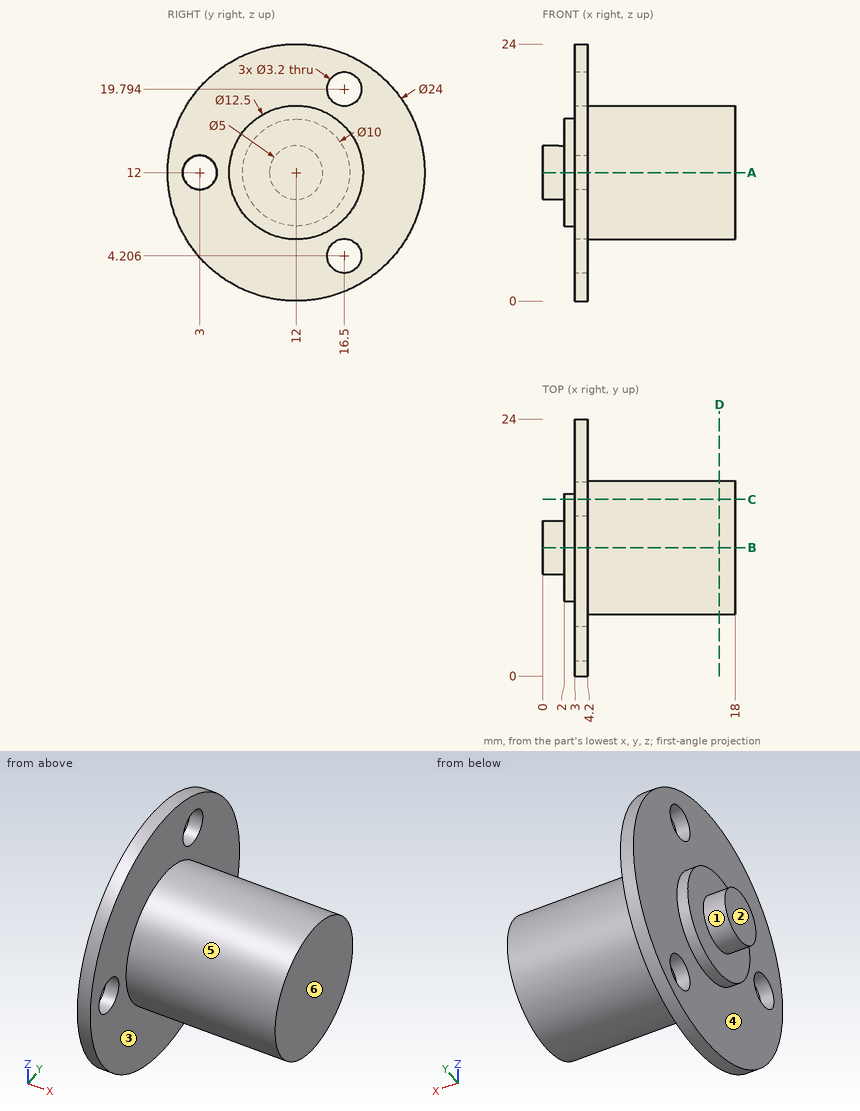
Drawing for the job (mm, zero at the part's lowest x, y, z). A direction names the side the tool comes from. Give positions to 0.01 mm unless a question says otherwise; leave off trailing zeros. Loops run counter-clockwise (first coordinate to the right, second up) from the corner with the lowest first, then second, coordinate; pieces in that order, holes last.
(1) Pull direction X, two halves, no side cores. Call the marked faces 4, 5 and 6: pulls with the +X half, pulls with the -X half, needs draft (parallel to the pull), parting line crosses it, or undercut.
Return value:
face 4: pulls with the -X half
face 5: needs draft
face 6: pulls with the +X half
(2) Band-saw the part on C-C (y = 16.5). Write the cut outline in (x, z), and give its area (3 significant figures).
Return value:
outline: (2, 9.82) - (3, 9.82) - (3, 5.81) - (4.2, 5.81) - (4.2, 7.66) - (18, 7.66) - (18, 16.34) - (4.2, 16.34) - (4.2, 18.19) - (3, 18.19) - (3, 14.18) - (2, 14.18) - close; (3, 0.88) - (4.2, 0.88) - (4.2, 2.61) - (3, 2.61) - close; (3, 21.39) - (4.2, 21.39) - (4.2, 23.12) - (3, 23.12) - close
area: 143 mm2
(3) Band-saw the part on A-A (z = 12). Write the cut outline in (x, y), and give its area (3 significant figures).
Return value:
outline: (0, 9.5) - (2, 9.5) - (2, 7) - (3, 7) - (3, 4.6) - (4.2, 4.6) - (4.2, 5.75) - (18, 5.75) - (18, 18.25) - (4.2, 18.25) - (4.2, 24) - (3, 24) - (3, 17) - (2, 17) - (2, 14.5) - (0, 14.5) - close; (3, 0) - (4.2, 0) - (4.2, 1.4) - (3, 1.4) - close
area: 217 mm2
(4) Pin check, flat tips, straight feed: pin 1 (4 mm diameter, centred on y = 16.5, z = 3, fed in from -X); pin 2 (6 mm diameter, centred on x = 13.5, z = 19.5, fed in from +Y); pin 3 (3 mm diameter, centred on x = 2.5, y = 19.5, fed in from -Z). Stop position of each tip, or through.
Return value:
pin 1: stops at x = 3
pin 2: stops at y = 16.34
pin 3: stops at z = 1.66
(5) Band-saw the part on D-D (x = 16.5). Write the cut outline in (y, z).
Return value:
outline: circle Ø12.5 at (12, 12)
(6) 3-axis set-ups, long thin cutter, end or side, ignore diameter. For the marked faces 1, 2 and 3: which of +Z, -Z, +X, -X, +Y, -Y reach the whole face in a straight line?
Return value:
face 1: -X
face 2: +Z, -Z, -X, +Y, -Y
face 3: +X
(7) Drill centre lines: line 1 along X through (y, z) = (19.5, 9); line 2 along Z through (x, y) = (7, 12); line 3 along Y through (x, z) = (3.5, 21). Where is each one in solid material? Low to high.
Return value:
line 1: x = 3 to 4.2
line 2: z = 5.75 to 18.25
line 3: y = 4.06 to 15.45, 17.55 to 19.94
(8) Band-saw the part on B-B (y = 12). Write the cut outline in (x, z).
Return value:
outline: (0, 9.5) - (2, 9.5) - (2, 7) - (3, 7) - (3, 0) - (4.2, 0) - (4.2, 5.75) - (18, 5.75) - (18, 18.25) - (4.2, 18.25) - (4.2, 24) - (3, 24) - (3, 17) - (2, 17) - (2, 14.5) - (0, 14.5) - close
